from build123d import *

# Parameters (mm, degrees)
BOX003_W     = 4.9
BOX003_H     = 12.4
BOX003_DEPTH = 10
BOX002_W     = 4.9
BOX002_H     = 12.4
BOX002_DEPTH = 10
BOX001_W     = 4.9
BOX001_H     = 12.4
BOX001_DEPTH = 10
BOX_W        = 52
BOX_H        = 20
BOX_DEPTH    = 15


with BuildPart() as cube003:
    # Box003 → Box003 (new body)
    with BuildSketch(Plane(origin=(43.5, 3, 6), x_dir=(1, 0, 0), z_dir=(0, 0, 1))):
        with Locations((2.45, 6.2)):
            Rectangle(BOX003_W, BOX003_H)
    extrude(amount=BOX003_DEPTH)


with BuildPart() as cube002:
    # Box002 → Box002 (new body)
    with BuildSketch(Plane(origin=(23.5, 3, 6), x_dir=(1, 0, 0), z_dir=(0, 0, 1))):
        with Locations((2.45, 6.2)):
            Rectangle(BOX002_W, BOX002_H)
    extrude(amount=BOX002_DEPTH)


with BuildPart() as cube001:
    # Box001 → Box001 (new body)
    with BuildSketch(Plane(origin=(3.5, 3, 6), x_dir=(1, 0, 0), z_dir=(0, 0, 1))):
        with Locations((2.45, 6.2)):
            Rectangle(BOX001_W, BOX001_H)
    extrude(amount=BOX001_DEPTH)


with BuildPart() as cut002:
    # Box → Box (new body)
    with BuildSketch(Plane.XY):
        with Locations((26, 10)):
            Rectangle(BOX_W, BOX_H)
    extrude(amount=BOX_DEPTH)

    # Cut: cut Cube001
    add(cube001.part, mode=Mode.SUBTRACT)

    # Cut001: cut Cube002
    add(cube002.part, mode=Mode.SUBTRACT)

    # Cut002: cut Cube003
    add(cube003.part, mode=Mode.SUBTRACT)


solid = cut002.part
Model file for the job. Use its own axes, mm. A direction names the side the tool comes from. Give positions to 0.01 mm unless a question says otherwise; leave off trailing zeros. Loops run counter-clockwise (first coordinate to the right, second up) from the corner with the lowest first, then second, coordinate; pieces in that order, holes last.
1) Saw through at C-C (y = 4.75). Write the cut outline in (x, z).
2) Wall check: line 1 (X direction, y = 11.5, z = 9); line 2 (Y direction, x = 25.5, z = 13.75); line 3 (Z direction, x = 47, y = 14.25). Give the ranges that are in metal, low to high.
3) Flat gauge pin, fed straight in: pin 1 Ø2.5 at (x, y) = (47, 11.5) entering from +Z. Where does the tip first touch, or does it go through?
4) Saw through at B-B (x = 46). Write the cut outline in (y, z), plus the area to 3 significant figures.
5) Saw through at A-A (z = 8). Write the cut outline in (x, y), plus the area to 3 significant figures.
6) Tool access for faces 1 (the flat face through (43.5, 9, 10)), 2 (the flat face through (0, 10, 7)): list every direction of +Z, -Z, +X, -X, +Y, -Y with a clear straight run to the whole face (end or side of a thin tool).
Answer block:
1. outline: (0, 0) - (52, 0) - (52, 15) - (48.4, 15) - (48.4, 6) - (43.5, 6) - (43.5, 15) - (28.4, 15) - (28.4, 6) - (23.5, 6) - (23.5, 15) - (8.4, 15) - (8.4, 6) - (3.5, 6) - (3.5, 15) - (0, 15) - close
2. line 1: x = 0 to 3.5, 8.4 to 23.5, 28.4 to 43.5, 48.4 to 52
2. line 2: y = 0 to 3, 15.4 to 20
2. line 3: z = 0 to 6
3. pin 1: stops at z = 6
4. outline: (0, 0) - (20, 0) - (20, 15) - (15.4, 15) - (15.4, 6) - (3, 6) - (3, 15) - (0, 15) - close
4. area: 188 mm2
5. outline: (0, 0) - (52, 0) - (52, 20) - (0, 20) - close; hole (3.5, 3) - (8.4, 3) - (8.4, 15.4) - (3.5, 15.4) - close; hole (23.5, 3) - (28.4, 3) - (28.4, 15.4) - (23.5, 15.4) - close; hole (43.5, 3) - (48.4, 3) - (48.4, 15.4) - (43.5, 15.4) - close
5. area: 858 mm2
6. face 1: +Z
6. face 2: +Z, -Z, -X, +Y, -Y
